from build123d import *

# Parameters (mm, degrees)
SKETCH1_R           = 1.9939
BOSS_EXTRUDE1_DEPTH = 5.9944
SKETCH2_R           = 2.5019
BOSS_EXTRUDE2_DEPTH = 3.9878
SKETCH3_R           = 1.9685
CUT_EXTRUDE1_DEPTH  = 10.9822
SKETCH4_W           = 1.99898
SKETCH4_H           = 3.683
CUT_EXTRUDE2_DEPTH  = 6.0038
CUT_EXTRUDE3_REACH  = 7.004
CUT_EXTRUDE4_REACH  = 7.004


with BuildPart() as part:
    # Sketch1 → Boss-Extrude1 (new body)
    with BuildSketch(Plane(origin=(0, 0, 0), x_dir=(1, 0, 0), z_dir=(0, 1, 0))):
        Circle(SKETCH1_R)
    extrude(amount=BOSS_EXTRUDE1_DEPTH)

    # Sketch2 → Boss-Extrude2 (add)
    with BuildSketch(Plane(origin=(0, 0, 0), x_dir=(1, 0, 0), z_dir=(0, 1, 0))):
        Circle(SKETCH2_R)
    extrude(amount=-BOSS_EXTRUDE2_DEPTH)

    # Sketch3 → Cut-Extrude1 (cut, through all)
    with BuildSketch(Plane(origin=(0, 5.9944, 0), x_dir=(1, 0, 0), z_dir=(0, 1, 0))):
        Circle(SKETCH3_R)
    extrude(amount=-CUT_EXTRUDE1_DEPTH, mode=Mode.SUBTRACT)

    # Sketch4 → Cut-Extrude2 (cut, through all)
    with BuildSketch(Plane.XY.offset(2.5019)):
        with Locations((-0.00381, -2.1463)):
            Rectangle(SKETCH4_W, SKETCH4_H)
    extrude(amount=-CUT_EXTRUDE2_DEPTH, mode=Mode.SUBTRACT)

    # Sketch6 → Cut-Extrude3 (cut, up to next)
    with BuildSketch(Plane(origin=(-2.5019, 0, 0), x_dir=(0, 0, -1), z_dir=(1, 0, 0)), mode=Mode.PRIVATE) as cut_extrude3_sk1:
        with BuildLine():
            Line((-2.295239627, -3.9878), (2.295239627, -3.9878))
            ThreePointArc((2.295239627, -3.9878), (1.432460388, -3.48008017), (0.463371203, -3.731145085))
            Line((0.463371203, -3.731145085), (0, -2.771398111))
            Line((0, -2.771398111), (-0.439998736, -3.731145085))
            ThreePointArc((-0.439998736, -3.731145085), (-1.420774155, -3.475239573), (-2.295239627, -3.9878))
        make_face()
    cut_extrude3_tool1 = extrude(cut_extrude3_sk1.sketch, amount=CUT_EXTRUDE3_REACH, mode=Mode.PRIVATE) & part.part
    add(cut_extrude3_tool1.solids().sort_by_distance((-2.5019, -3.705676, 0.002257))[0], mode=Mode.SUBTRACT)

    # Sketch5 → Cut-Extrude4 (cut, up to next)
    with BuildSketch(Plane(origin=(2.5019, 0, 0), x_dir=(0, 0, -1), z_dir=(1, 0, 0)), mode=Mode.PRIVATE) as cut_extrude4_sk1:
        with BuildLine():
            Line((0.463371203, -3.731145085), (0, -2.771398111))
            Line((0, -2.771398111), (-0.439998736, -3.731145085))
            ThreePointArc((-0.439998736, -3.731145085), (-1.420774155, -3.475239573), (-2.295239627, -3.9878))
            Line((-2.295239627, -3.9878), (2.295239627, -3.9878))
            ThreePointArc((2.295239627, -3.9878), (1.432460388, -3.48008017), (0.463371203, -3.731145085))
        make_face()
    cut_extrude4_tool1 = extrude(cut_extrude4_sk1.sketch, amount=-CUT_EXTRUDE4_REACH, mode=Mode.PRIVATE) & part.part
    add(cut_extrude4_tool1.solids().sort_by_distance((2.5019, -3.705676, 0.002257))[0], mode=Mode.SUBTRACT)


solid = part.part
Verification items for the finished model (mm, model axes). Give positions to 0.01 mm unless a question says otherwise; leave off trailing zeros. Order: outer loops, then holes, each group sorted by start corner. A loop starts at its lowest first (then second) coordinate and runs counter-clockwise, first axis right, second up. Notation, with made-up numbers: M 27.25,77 L 43.25,77 A22 cw 43.25,83 Z; hole C 43,68 d3. An arc over 180 degrees is marked long. Use one line per item in the form item = value. Start each with the question number.
Q1. Scan lines: line 1 along Z through (x, y) = (1.6, -1.5); line 2 along X through (y, z) = (-3.5, 2.2); line 3 along X through (y, z) = (-2, 1.95). Record each from-to range of solid material in increasing order. Write a range as [from, to].
Q2. Mould release check, pull along X, two halves, no side actions. Record for faces 1 (the flat face through (0, -0.305, -2.2)), 2 (the cylindrical face through (2.386, -1.523, -0.752)), 3 (the flat face through (0, -0.305, 2.2)), 4 (the flat face through (-2, 0, 1)): +X half, -X half, draft (parallel to the pull), parting line (faces both ways), or undercut.
Q3. Section check B-B (y = -2.25). Enter the section's corners in (x, z), then the cut area to 3 significant figures.
Q4. Go/stop test with flat-tipped pins: pin 1 Ø2 at (y, z) = (0.5, -1) entering from +X; pin 2 Ø0.5 at (y, z) = (-1.5, 2) entering from -X; pin 3 Ø0.5 at (y, z) = (-2, -2) entering from +X. Record where each tip stops, or that it passes through.
Q5. Section check D-D (y = 2.5). Enter the section's corners in (x, z).
Evaluation:
q1.line_1 = [-1.92, -1.15], [1.15, 1.92]
q1.line_2 = [-1.19, -1], [1, 1.19]
q1.line_3 = [-1.57, -1], [1, 1.57]
q2.face_1 = undercut
q2.face_2 = parting line
q2.face_3 = undercut
q2.face_4 = draft
q3.outline = M -1,-2.29 L -1,-1.69 A1.97 cw -1,1.69 L -1,2.29 A2.5 ccw Z; M 1,-2.3 A2.5 ccw 1,2.3 L 1,1.7 A1.97 cw 1,-1.7 Z
q3.area = 5.28 mm2
q4.pin_1 = 2.5
q4.pin_2 = -1.79
q4.pin_3 = 1.79
q5.outline = C 0,0 d3.99; hole C 0,0 d3.94
